```python
from build123d import *

# Parameters (mm, degrees)
F1_DEPTH = 2
F2_R     = 0.5


with BuildPart() as f1:
    # F0 (on Top) → F1 (new body)
    with BuildSketch(Plane.XY):
        Polygon((1.5, 1.875), (1.5, 1.85), (2.5, 1.85), (2.5, 3.85), (0.5, 3.85), (0.5, 3.35), (-0.5, 3.35), (-0.5, 3.85), (-2.5, 3.85), (-2.5, 1.85), (-1.5, 1.85), (-1.5, 1.875), align=None)
        Polygon((1.5, 1.85), (1.5, -1.875), (-1.5, -1.875), (-1.5, 1.85), (-2.5, 1.85), (-5, 1.85), (-5, -3.15), (5, -3.15), (5, 1.85), (2.5, 1.85), align=None)
    extrude(amount=F1_DEPTH)

    # F2
    f2_edges = [f1.edges().sort_by_distance(p)[0] for p in [
        (-2.5, 3.85, 1),
        (2.5, 3.85, 1),
    ]]
    fillet(f2_edges, radius=F2_R)


solid = f1.part
```
Here's how the part is built. I have some questions about the finished solid (model axes, mm). A direction names the side the tool comes from. Coordinates: 2 decimals unless noted, no trailing zeros. Write each loop counter-clockwise with the first axis right and the second up, starting at its lowest first coordinate (ties: lowest second). Pieces come first, ordered by that corner, then holes. Notation, with made-up numbers: (80.25, -35) - (121.25, -35) arc R15 cw to (121.25, -8) - close; hole circle Ø6 at (35, 66). An arc over 180 degrees is marked (long way). One line per item, written item: value.
1) I'm going to push flat-ended pins straight in: P1, Ø0.8, axis at x = 0, z = 0.5, coming from the +Y side; P2, Ø1.5, axis at x = 3.5, y = 2.5, coming from the +Z side; P3, Ø1.2, axis at y = 2.5, z = 0.5, coming from the -X side; P4, Ø1.2, axis at y = 2.5, z = 1, coming from the +X side. Where does each tip first touch, or does it pass through?
Model answer:
P1: stops at y = 3.35
P2: stops at z = 2
P3: stops at x = -2.5
P4: stops at x = 2.5
2) I need wall thicknesses on line 1 along X through (y, z) = (0, 0.85); line 2 along Y through (x, z) = (-1, 1.8) (3 decimals); line 3 along Y through (x, z) = (-4, 1.2). Which ranges of each line are inside material? Lowest first, please.
Model answer:
line 1: x = -5 to -1.5, 1.5 to 5
line 2: y = -3.15 to -1.875, 1.875 to 3.85
line 3: y = -3.15 to 1.85
3) Suppose I cut it at B-B on x = 0. Write out the boundary of the cut face in (y, z) (3 decimals), and give its area (3 significant figures).
Model answer:
outline: (-3.15, 0) - (-1.875, 0) - (-1.875, 2) - (-3.15, 2) - close; (1.875, 0) - (3.35, 0) - (3.35, 2) - (1.875, 2) - close
area: 5.50 mm²
4) On a 3-axis mill with a long thin cutter (end or side, diameter ignored), from which of +Z, -Z, +X, -X, +Y, -Y can I reach the whole of each face in a straight line? I mean faces 4 (the flat face through (0, 3.35, 1)), 5 (the flat face through (4, 1.85, 1)), 6 (the flat face through (0, 1.875, 1)). Say none if no direction works.
Model answer:
face 4: +Z, -Z, +Y
face 5: +Z, -Z, +X, +Y
face 6: +Z, -Z
5) Suppose I cut it at A-A on y = -0.25. Write out the boundary of the cut face in (x, z).
Model answer:
outline: (-5, 0) - (-1.5, 0) - (-1.5, 2) - (-5, 2) - close; (1.5, 0) - (5, 0) - (5, 2) - (1.5, 2) - close
6) We'd pull the mould along X, two halves only. Please class faces 1 (the flat face through (-2, 0, 2)), 2 (the flat face through (-2.5, 3, 1)), 3 (the flat face through (-1.5, 0, 1)): pulls with the +X half, pulls with the -X half, needs draft (parallel to the pull), parting line crosses it, or undercut.
Model answer:
face 1: needs draft
face 2: pulls with the -X half
face 3: undercut
7) Suppose I cut it at C-C on z = 0.85. Write out the boundary of the cut face in (x, y) (3 decimals), and give its area (3 significant figures).
Model answer:
outline: (-5, -3.15) - (5, -3.15) - (5, 1.85) - (2.5, 1.85) - (2.5, 3.35) arc R0.5 ccw to (2, 3.85) - (0.5, 3.85) - (0.5, 3.35) - (-0.5, 3.35) - (-0.5, 3.85) - (-2, 3.85) arc R0.5 ccw to (-2.5, 3.35) - (-2.5, 1.85) - (-5, 1.85) - close; hole (-1.5, -1.875) - (1.5, -1.875) - (1.5, 1.875) - (-1.5, 1.875) - close
area: 48.1 mm²
8) Suppose I cut it at D-D on y = 2.75. Write out the boundary of the cut face in (x, z).
Model answer:
outline: (-2.5, 0) - (2.5, 0) - (2.5, 2) - (-2.5, 2) - close
